from build123d import *

# Parameters (mm, degrees)
CROQUIS1_R              = 35
CROQUIS1_R_2            = 25
SALIENTE_EXTRUIR1_DEPTH = 2
CROQUIS2_R              = 27.1
CROQUIS2_R_2            = 26.1
SALIENTE_EXTRUIR3_DEPTH = 15
CROQUIS5_R              = 2.5
SALIENTE_EXTRUIR5_DEPTH = 18.5


with BuildPart() as part:
    # Croquis1 → Saliente-Extruir1 (new body)
    with BuildSketch(Plane.XY):
        Circle(CROQUIS1_R)
        Circle(CROQUIS1_R_2, mode=Mode.SUBTRACT)
    extrude(amount=SALIENTE_EXTRUIR1_DEPTH)

    # Croquis2 → Saliente-Extruir3 (add)
    with BuildSketch(Plane(origin=(0, 0, 0), x_dir=(-1, 0, 0), z_dir=(0, 0, -1))):
        with Locations(Location((0, 0, 0), (0, 0, 180))):
            Circle(CROQUIS2_R)
        Circle(CROQUIS2_R_2, mode=Mode.SUBTRACT)
    extrude(amount=SALIENTE_EXTRUIR3_DEPTH)

    # Croquis5 → Saliente-Extruir5 (add)
    with BuildSketch(Plane(origin=(0, 0, 0), x_dir=(-1, 0, 0), z_dir=(0, 0, -1))):
        with Locations(Location((31.5, 0, 0), (0, 0, 180))):
            Circle(CROQUIS5_R)
        with Locations(Location((22.273863607, -22.273863607, 0), (0, 0, 180))):
            Circle(CROQUIS5_R)
        with Locations(Location((0, -31.5, 0), (0, 0, 180))):
            Circle(CROQUIS5_R)
        with Locations(Location((-22.273863607, -22.273863607, 0), (0, 0, 180))):
            Circle(CROQUIS5_R)
        with Locations(Location((-31.5, 0, 0), (0, 0, 180))):
            Circle(CROQUIS5_R)
        with Locations(Location((-22.273863607, 22.273863607, 0), (0, 0, 180))):
            Circle(CROQUIS5_R)
        with Locations(Location((0, 31.5, 0), (0, 0, 180))):
            Circle(CROQUIS5_R)
        with Locations(Location((22.273863607, 22.273863607, 0), (0, 0, 180))):
            Circle(CROQUIS5_R)
    extrude(amount=SALIENTE_EXTRUIR5_DEPTH)


solid = part.part
Check sheet for the modelled part. Datum: model origin and axes. Units: mm. A direction names the side the tool comes from. Give positions to 0.01 mm unless a question says otherwise; leave off trailing zeros. Order: outer loops, then holes, each group sorted by start corner. A loop starts at its lowest first (then second) coordinate and runs counter-clockwise, first axis right, second up. Notation, with made-up numbers: M 83.5,18 L 114.5,18 A18 ccw 114.5,52 Z; hole C -22,50.25 d3. An arc over 180 degrees is marked long. Answer as CSV lines item,"result". Start each with the question number.
Item 1: Gauge pin test, flat ends, axial feed: P1, Ø5, axis at y = -0.5, z = -3, coming from the -X side; P2, Ø3, axis at x = 20, z = -13, coming from the +Y side; P3, Ø12, axis at x = 15.5, z = -8, coming from the -Y side. Record the tip position at first contact, or that the pin passes through.
Item 2: Cross-section at D-D on y = -31.5. Enter the section's corners in (x, z).
Item 3: Mould release check, pull along X, two halves, no side actions. Record for faces 3 (the face through (-28, -21, 1)), 4 (the face through (22, 22, -18.5)), 5 (the face through (-24.116, 20.584, -9.12)): +X half, -X half, draft (parallel to the pull), parting line (faces both ways), or undercut.
Item 4: Thickness scan on line 1 (Y direction, x = 0, z = 0.85); line 2 (Y direction, x = -23.5, z = -3.25); line 3 (Y direction, x = -24, z = -12.25). Record the ranges inside material, lowest first. Write a range as [from, to].
Item 5: Cross-section at A-A on y = 0. Enter the section's corners in (x, z), plus the area to 3 significant figures.
Item 6: Cross-section at C-C on z = -7. State how many separate pieces and enclosed holes the cut face has, plus the area to 3 significant figures.
Item 7: Tool access check on faces 1 (the face through (12.505, 24.042, -7.395)), 2 (the face through (0, -32, -18.5)). Record the directions out of +Z, -Z, +X, -X, +Y, -Y that give a thin tool (end or side, any length) a straight path to the whole face; none if there is none.
Established:
1,P1,"stops at x = -34"
1,P2,"stops at y = 24.65"
1,P3,"stops at y = -25.38"
2,outline,"M -15.26,0 L -2.5,0 L -2.5,-18.5 L 2.5,-18.5 L 2.5,0 L 15.26,0 L 15.26,2 L -15.26,2 Z"
3,face 3,"parting line"
3,face 4,"draft"
3,face 5,"undercut"
4,line 1,"y = [-35, -25], [25, 35]"
4,line 2,"y = [-24.45, -20.1], [-13.5, -11.36], [11.36, 13.5], [20.1, 24.45]"
4,line 3,"y = [-24.08, -20.47], [-12.59, -10.26], [10.26, 12.59], [20.47, 24.08]"
5,outline,"M -35,0 L -34,0 L -34,-18.5 L -29,-18.5 L -29,0 L -27.1,0 L -27.1,-15 L -26.1,-15 L -26.1,0 L -25,0 L -25,2 L -35,2 Z; M 25,0 L 26.1,0 L 26.1,-15 L 27.1,-15 L 27.1,0 L 29,0 L 29,-18.5 L 34,-18.5 L 34,0 L 35,0 L 35,2 L 25,2 Z"
5,area,"255 mm^2"
6,separate pieces,"9"
6,enclosed holes,"1"
6,area,"324 mm^2"
7,face 1,"-Z"
7,face 2,"-Z, +X, -X, +Y, -Y"
